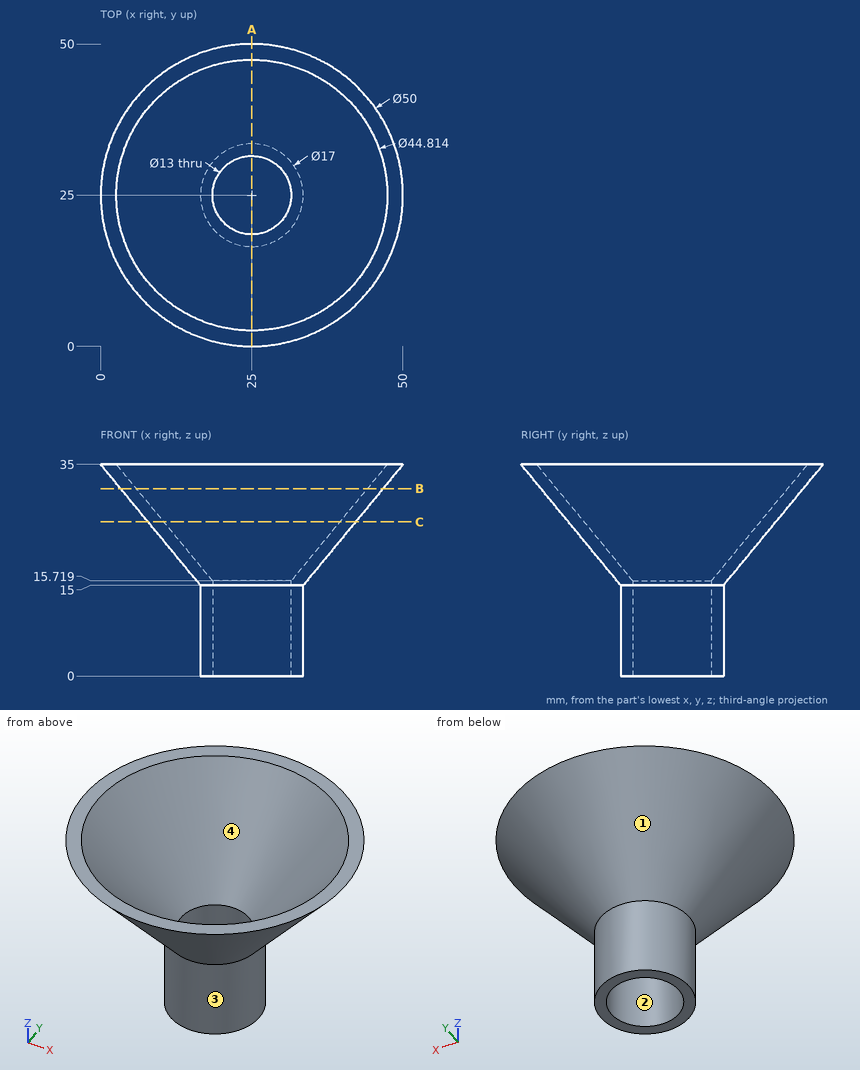
Can you work these out from the drawing? Everything is in mm from the part's minimum corner. A direction names the side the tool comes from. Coordinates: 2 decimals unless noted, no trailing zeros. Write each loop counter-clockwise with the first axis right and the second up, starting at its lowest first coordinate (ties: lowest second). Pieces come first, ordered by that corner, then holes. Notation, with made-up numbers: (-21.5, 87.25) - (1.5, 87.25) arc R23 cw to (1.5, 125.25) - close; hole circle Ø8 at (-9, 5). An arc over 180 degrees is marked (long way). One line per item, written item: value.
1) We'd pull the mould along X, two halves only. Please class the marked faces 1 and 2: pulls with the +X half, pulls with the -X half, needs draft (parallel to the pull), parting line crosses it, or undercut.
Model answer:
face 1: parting line crosses it
face 2: undercut
2) Suppose I cut it at A-A on x = 25. Write out the boundary of the cut face in (y, z).
Model answer:
outline: (0, 35) - (16.5, 15) - (16.5, 0) - (18.5, 0) - (18.5, 15.72) - (2.59, 35) - close; (31.5, 0) - (33.5, 0) - (33.5, 15) - (50, 35) - (47.41, 35) - (31.5, 15.72) - close
3) I need wall thicknesses on line 1 along Y through (x, z) = (25, 7.5); line 2 along Y through (x, z) = (19, 27) (1 decimal); line 3 along X through (y, z) = (31, 13.5) (1 decimal). Which ranges of each line are inside material? Lowest first, please.
Model answer:
line 1: y = 16.5 to 18.5, 31.5 to 33.5
line 2: y = 7.6 to 10.4, 39.6 to 42.4
line 3: x = 19 to 22.5, 27.5 to 31
4) I'm going to push flat-ended pins straight in: P1, Ø8, axis at y = 7.5, z = 27.5, coming from the +X side; P2, Ø1.5, axis at x = 28, z = 12.5, coming from the -Y side; P3, Ø8, axis at y = 29.5, z = 9.5, coming from the -X side (1 decimal). Where does each tip first touch, or does it pass through?
Model answer:
P1: stops at x = 40.25
P2: stops at y = 16.8
P3: stops at x = 16.5
5) Suppose I cut it at B-B on z = 31. Write out the boundary of the cut face in (x, y) (1 decimal).
Model answer:
outline: circle Ø43.4 at (25, 25); hole circle Ø38.2 at (25, 25)
6) Suppose I cut it at C-C on z = 25.5. Write out the boundary of the cut face in (x, y) (1 decimal).
Model answer:
outline: circle Ø34.3 at (25, 25); hole circle Ø29.1 at (25, 25)
7) On a 3-axis mill with a long thin cutter (end or side, diameter ignored), from which of +Z, -Z, +X, -X, +Y, -Y can I reach the whole of each face in a straight line? I mean the marked faces 3 and 4. Say none if no direction works.
Model answer:
face 3: -Z
face 4: +Z
